Geometry check sheet. Reference: the model listing, model coordinates, mm. A direction names the side the tool comes from. Give positions to 0.01 mm unless a question says otherwise; leave off trailing zeros. Loops run counter-clockwise (first coordinate to the right, second up) from the corner with the lowest first, then second, coordinate; pieces in that order, holes last. Notation, with made-up numbers: (26, 6) -> (48, 6) arc R14 cw to (48, 21) -> close; hole circle Ø7 at (48.5, 16.25). An arc over 180 degrees is marked (long way). One line per question, with ' | ' between items.
Autodesk Inventor part; units mm, degrees
ref_plane "YZ-Ebene" through (0, 0, 0) normal (1, 0, 0) x (0, 1, 0)
ref_plane "XZ-Ebene" through (0, 0, 0) normal (0, 1, 0) x (-1, 0, 0)
ref_plane "XY-Ebene" through (0, 0, 0) normal (0, 0, 1) x (1, 0, 0)
sketch "Skizze1" plane through (0, 0, 0) normal (0, 0, 1) x (1, 0, 0)
  line L0 (-12, 0) -> (2, 0)
  line L1 (0, -0.6) -> (0, 3.6)
  line L2 (0, 3) -> (-4, 3)
  line L3 (-4, 3) -> (-4, 2.5)
  line L4 (-4, 2.5) -> (-10, 2.5)
  line L5 (-10, 2.5) -> (-10, 1.25)
  line L6 (-10, 1.25) -> (-3.5, 1.25)
  line L7 (-3.5, 1.25) -> (-3.5, 0.5)
  line L8 (-3.5, 0.5) -> (0, 0.5)
  point P0 (0, 0)
  dimension "d1" = 6
  dimension "d2" = 1
  dimension "d3" = 5
  dimension "d4" = 2.5
  dimension "d5" = 6.5
  dimension "d6" = 4
  dimension "d7" = 10
revolve "Umdrehung1" add sketch "Skizze1" angle 360 about axis through (-10, 0, 0) along (1, 0, 0)
sketch "Skizze2" plane through (0, 0, 0) normal (1, 0, 0) x (0, 0, -1)
  line L0 (0, -4.2) -> (0, 4.2)
  line L1 (4.33, 0) -> (-4.98, 0)
  circle A0 centre (-3.25, 0) radius 0.4
  dimension "d11" = 0.8
  dimension "d12" = 6.5
extrude "Extrusion1" cut sketch "Skizze2" against normal blind 4
pattern_circular "Runde Anordnung1" count 22 over 360 about axis through (-10, 0, 0) along (1, 0, 0) of "Extrusion1"
thread "Gewinde1"
properties part number "Nadelhalter_ra8846s" material "Aluminium 6061"
Item 1: Scan lines: probe 1 along Z at (x, y) = (-2.05, 0); probe 2 along Z at (x, y) = (-8, 0); probe 3 along Z at (x, y) = (-3, 1.8). Record each from-to range of solid material in increasing order.
Result:
probe 1: -2.85 to -0.5, 0.5 to 2.85 | probe 2: -2.5 to -1.25, 1.25 to 2.5 | probe 3: -2.34 to 2.34
Item 2: Sectioned sample at C-C (z = 0.85). Record the cut outline in (x, y), plus the area to 3 significant figures.
Result:
outline: (-10, -2.35) -> (-4, -2.35) -> (-4, -2.88) -> (0, -2.88) -> (0, 2.88) -> (-4, 2.88) -> (-4, 2.35) -> (-10, 2.35) -> (-10, 0.92) -> (-3.5, 0.92) -> (-3.5, -0.92) -> (-10, -0.92) -> close | area: 39.3 mm2
Item 3: Depth check by flat-ended pin: pin 1 Ø3 at (y, z) = (0.5, -0.5) entering from -X. Enter the tip coordinate at first touch or a pass-through.
Result:
pin 1: x = -10
Item 4: Release check for a two-part mould opening along Y. For faces 1 (the face through (-6.7, -0.27, -1.22)), 2 (the face through (-10, 1, 1)), 3 (the face through (-7.04, -0.54, 2.44)) record: pulls with the +Y half, pulls with the -Y half, needs draft (parallel to the pull), parting line crosses it, or undercut.
Result:
face 1: undercut | face 2: needs draft | face 3: parting line crosses it
Item 5: Sectioned sample at B-B (z = 0). Record the cut outline in (x, y).
Result:
outline: (-10, -2.5) -> (-4, -2.5) -> (-4, -3) -> (0, -3) -> (0, -0.5) -> (-3.5, -0.5) -> (-3.5, -1.25) -> (-10, -1.25) -> close; (-10, 1.25) -> (-3.5, 1.25) -> (-3.5, 0.5) -> (0, 0.5) -> (0, 3) -> (-4, 3) -> (-4, 2.5) -> (-10, 2.5) -> close
Item 6: Set-up check for faces 4 (the face through (0, 0, -1)), 5 (the face through (-3.5, 1, 0)): record each of +Z, -Z, +X, -X, +Y, -Y from which the full face is reachable in a straight line by a thin tool's end or side.
Result:
face 4: +Z, -Z, +X, +Y, -Y | face 5: -X
Item 7: Sectioned sample at D-D (x = -8.25). Record the cut outline in (y, z).
Result:
outline: circle Ø5 at (0, 0); hole circle Ø2.5 at (0, 0)
Item 8: Sectioned sample at A-A (y = 0). Record the cut outline in (x, z), plus the area to 4 significant figures.
Result:
outline: (-10, -2.5) -> (-4, -2.5) -> (-4, -2.85) -> (0, -2.85) -> (0, -0.5) -> (-3.5, -0.5) -> (-3.5, -1.25) -> (-10, -1.25) -> close; (-10, 1.25) -> (-3.5, 1.25) -> (-3.5, 0.5) -> (0, 0.5) -> (0, 2.85) -> (-4, 2.85) -> (-4, 2.5) -> (-10, 2.5) -> close | area: 33.05 mm2
